Geometry check sheet. Reference: the model listing, model coordinates, mm. A direction names the side the tool comes from. Give positions to 0.01 mm unless a question says otherwise; leave off trailing zeros. Write each loop counter-clockwise with the first axis right and the second up, starting at its lowest first coordinate (ties: lowest second). Pieces come first, ordered by that corner, then holes. Notation, with made-up numbers: (58.25, 80) - (111.25, 80) arc R19 cw to (111.25, 112) - close; hole circle Ø3 at (-28.75, -14). An arc over 180 degrees is marked (long way). Use a Markdown table: item, result.
```python
from build123d import *

# Parameters (mm, degrees)
F2_DEPTH = 2.5
F3_COUNT = 2
F3_ANGLE = 30


with BuildPart() as f1:
    # F0 (on Front) → F1 (revolve)
    with BuildSketch(Plane.XZ):
        Polygon((-71.3012740016, 0), (0, 0), (0, 41.3423627615), (-71.3012740016, 41.3423627615), (-71.3012740016, 32.3902414565), (-51.2194111943, 28.151858598), (-52.2884099565, 23.0868403589), (-71.3012740016, 27.0996054014), align=None)
        Polygon((-71.3012740016, 32.3902414565), (-71.3012740016, 27.0996054014), (-52.2884099565, 23.0868403589), (-51.2194111943, 28.151858598), align=None)
    revolve(axis=Axis((0, 0, 20.6711813807), (0, 0, 1)))

    # F0 (on Front) → F2 (join, symmetric)
    with BuildSketch(Plane.XZ):
        Polygon((-120.9029449902, 37.5682991719), (-71.3012740016, 27.0996054014), (-71.3012740016, 32.3902414565), (-119.833946228, 42.6333174109), align=None)
        Polygon((-71.3012740016, 32.3902414565), (-71.3012740016, 27.0996054014), (-52.2884099565, 23.0868403589), (-51.2194111943, 28.151858598), align=None)
    f2 = extrude(amount=F2_DEPTH, both=True)

    # F3: F2 ×2 about axis
    f3_axis = Axis((0, 0, 41.3423627615), (0, 0, -1))
    for i in range(1, F3_COUNT):
        add(f2.rotate(f3_axis, i * F3_ANGLE / (F3_COUNT - 1)))


solid = f1.part
```
1) Section check C-C on y = 13.5. Record the boundary of the cut face in (x, z).
Working result:
| item | result |
|---|---|
| outline | (-70.01, 0) - (70.01, 0) - (70.01, 41.34) - (-70.01, 41.34) - close |
2) Section check B-B on x = 0. Record the boundary of the cut face in (y, z), then the cut area to 3 significant figures.
Working result:
| item | result |
|---|---|
| outline | (-71.3, 0) - (71.3, 0) - (71.3, 41.34) - (-71.3, 41.34) - close |
| area | 5,900 mm² |
3) Depth check by flat-ended pin: P1, Ø6, axis at x = 39, z = 38.5, coming from the -Y side; P2, Ø12, axis at x = 22, y = 51.5, coming from the +Z side; P3, Ø12, axis at x = 0.5, z = 36.5, coming from the +Y side. Enter the tip coordinate at first touch or a pass-through.
Working result:
| item | result |
|---|---|
| P1 | stops at y = -61.55 |
| P2 | stops at z = 41.34 |
| P3 | stops at y = 71.3 |
4) Set-up check for faces 5 (the flat face through (-96, 2.5, 35)), 6 (the flat face through (-82.058, 50.263, 34.898)), 7 (the flat face through (-1, -1, 41.342)): record each of +Z, -Z, +X, -X, +Y, -Y from which the full face is reachable in a straight line by a thin tool's end or side.
Working result:
| item | result |
|---|---|
| face 5 | +Z, -Z, -X |
| face 6 | +Z, -Z, +Y |
| face 7 | +Z, +X, +Y, -Y |
5) Mould release check, pull along X, two halves, no side actions. Record for faces 1 (the flat face through (-82.468, 47.573, 37.435)), 2 (the flat face through (-95.206, -0.035, 37.435)), 3 (the flat face through (-96, -2.5, 35)), 4 (the flat face through (-84.558, 45.933, 34.898)): pulls with the +X half, pulls with the -X half, needs draft (parallel to the pull), parting line crosses it, or undercut.
Working result:
| item | result |
|---|---|
| face 1 | undercut |
| face 2 | undercut |
| face 3 | needs draft |
| face 4 | pulls with the -X half |
6) Material ranges on L1, parallel to Z at x = -66, y = 19; L2, parallel to Y at x = 1, z = 14; L3, parallel to X at y = -51, z = 13.5, recorded low to high. Write a range as from..to.
Working result:
| item | result |
|---|---|
| L1 | z = 0..41.34 |
| L2 | y = -71.29..71.29 |
| L3 | x = -49.83..49.83 |
7) Section check A-A on z = 14.5. Record the boundary of the cut face in (x, y).
Working result:
| item | result |
|---|---|
| outline | circle Ø142.6 at (0, 0) |
